Can you work these out from the model? Positions are in its coordinate system, mm. A direction names the side the tool comes from. Coordinates: 2 decimals unless noted, no trailing zeros. Write each loop counter-clockwise with the first axis right and the second up, starting at its lowest first coordinate (ties: lowest second). Pieces come first, ordered by that corner, then holes. Notation, with made-up numbers: (77, 6.5) -> (120, 6.5) arc R15 cw to (120, 11.5) -> close; hole circle Ø3 at (-14, 6.25). An arc over 180 degrees is marked (long way). Use one line per item in the form item = value.
```python
from build123d import *

# Parameters (mm, degrees)
SKETCH_1_R          = 6
EXTRUDE_1_DEPTH     = 6
CUT_EXTRUDE_START   = -6
CUT_EXTRUDE_1_DEPTH = 6
FILLET_1_R          = 6
SKETCH_6_R          = 1.5
CUT_EXTRUDE_2_DEPTH = 10
SKETCH_7_R          = 6
CUT_EXTRUDE_3_DEPTH = 10
FILLET_2_R          = 3


with BuildPart() as part:
    # 草图1 → 凸台-拉伸1 (new body)
    with BuildSketch(Plane.XY):
        with BuildLine():
            Line((0, 12), (150, 12))
            ThreePointArc((150, 12), (162, 0), (150, -12))
            Line((150, -12), (0, -12))
            ThreePointArc((0, -12), (-12, 0), (0, 12))
        make_face()
        Circle(SKETCH_1_R, mode=Mode.SUBTRACT)
        with Locations((150, 0)):
            Circle(SKETCH_1_R, mode=Mode.SUBTRACT)
    extrude(amount=EXTRUDE_1_DEPTH)

    # 草图2 → 切除-拉伸1 (cut)
    with BuildSketch(Plane.XY.offset(6).offset(CUT_EXTRUDE_START)):
        with BuildLine():
            ThreePointArc((10.908712115, -5), (6.480740698, -10.099504938), (0, -12))
            Line((0, -12), (150, -12))
            ThreePointArc((150, -12), (143.519259302, -10.099504938), (139.091287885, -5))
            Line((139.091287885, -5), (10.908712115, -5))
        make_face()
    extrude(amount=CUT_EXTRUDE_1_DEPTH, mode=Mode.SUBTRACT)

    # 圆角1
    fillet_1_edges = [part.edges().sort_by_distance(p)[0] for p in [
        (139.091287885, -5, 3),
        (10.908712115, -5, 3),
    ]]
    fillet(fillet_1_edges, radius=FILLET_1_R)

    # 草图6 → 切除-拉伸2 (cut)
    with BuildSketch(Plane.XY.offset(6)):
        with Locations((15, 1)):
            Circle(SKETCH_6_R)
        with Locations((35, 1)):
            Circle(SKETCH_6_R)
        with Locations((55, 1)):
            Circle(SKETCH_6_R)
        with Locations((75, 1)):
            Circle(SKETCH_6_R)
        with Locations((95, 1)):
            Circle(SKETCH_6_R)
        with Locations((115, 1)):
            Circle(SKETCH_6_R)
        with Locations((135, 1)):
            Circle(SKETCH_6_R)
    extrude(amount=-CUT_EXTRUDE_2_DEPTH, mode=Mode.SUBTRACT)

    # 草图7 → 切除-拉伸3 (cut)
    with BuildSketch(Plane(origin=(0, 0, 0), x_dir=(-1, 0, 0), z_dir=(0, 0, -1))):
        with Locations((-131.694159211, -9.484293539)):
            Circle(SKETCH_7_R)
    extrude(amount=-CUT_EXTRUDE_3_DEPTH, mode=Mode.SUBTRACT)

    # 圆角2
    fillet_2_edges = [part.edges().sort_by_distance(p)[0] for p in [
        (127.707793516, -5, 3),
        (135.680524907, -5, 3),
    ]]
    fillet(fillet_2_edges, radius=FILLET_2_R)


solid = part.part
```
Q1. Suppose I cut it at B-B (y = 4). Write out the boundary of the cut face in (x, z), then the cut area to 3 significant figures.
Return value:
outline = (-11.31, 0) -> (-4.47, 0) -> (-4.47, 6) -> (-11.31, 6) -> close; (4.47, 0) -> (145.53, 0) -> (145.53, 6) -> (4.47, 6) -> close; (154.47, 0) -> (161.31, 0) -> (161.31, 6) -> (154.47, 6) -> close
area = 928 mm2
Q2. If I drill on line 1 (X direction, y = 2.75, z = 2.5); line 2 (Y direction, x = 15, z = 4.65); line 3 (X direction, y = -5.5, z = 0.75), over which ranges is the centre line in solid material (lowest first)? Write a range as from..to.
Return value:
line_1 = -11.68..-5.33, 5.33..144.67, 155.33..161.68
line_2 = -5..-0.5, 2.5..12
line_3 = -10.67..-2.4, 2.4..11.85, 138.15..147.6, 152.4..160.67
Q3. Thinking about a two-plate mould opening in X: for faces 1 (the flat face through (74, 12, 3)), 2 (the cylindrical face through (138.73, -5.79, 3.04)), which applies, released by +X, released by -X, zero draft, split by the parting line, or undercut?
Return value:
face_1 = zero draft
face_2 = undercut
Q4. Suppose I cut it at D-D (y = 10.25). Write out the boundary of the cut face in (x, z), then the cut area to 3 significant figures.
Return value:
outline = (-6.24, 0) -> (156.24, 0) -> (156.24, 6) -> (-6.24, 6) -> close
area = 975 mm2
Q5. Suppose I cut it at C-C (z = 2). Give the number of separate pieces and of enclosed holes in the cut face, then the cut area to 3 significant figures.
Return value:
separate_pieces = 1
enclosed_holes = 9
area = 2,830 mm2
Q6. Will these pins go through, and if not, where does the flat tip stop? pin 1 (9.5 mm diameter, centred on x = 150, y = 0, fed in from +Z); pin 2 (8 mm diameter, centred on x = 10.5, y = -8.5, fed in from +Z); pin 3 (2 mm diameter, centred on y = -2.5, z = 1, fed in from -X).
Return value:
pin_1 = through
pin_2 = 6
pin_3 = -11.91
Q7. Suppose I cut it at A-A (x = 95). Write out the boundary of the cut face in (y, z), then the cut area to 3 significant figures.
Return value:
outline = (-5, 0) -> (-0.5, 0) -> (-0.5, 6) -> (-5, 6) -> close; (2.5, 0) -> (12, 0) -> (12, 6) -> (2.5, 6) -> close
area = 84.0 mm2
Q8. For faces 3 (the flat face through (71, -5, 3)), 4 (the cylindrical face through (76.43, 1.45, 3.04)), which set-ups out of +Z, -Z, +X, -X, +Y, -Y let a thin tool reach every point of the face, with its end or its side?
Return value:
face_3 = +Z, -Z, -Y
face_4 = +Z, -Z
